from build123d import *

# Parameters (mm, degrees)
SKETCH2_R                 = 2.5
BOSS_EXTRUDE1_DEPTH       = 18
FILLET3_R                 = 1
BOSS_EXTRUDE2_START       = -1
SKETCH5_R                 = 3.75
SKETCH5_R_2               = 2.5
BOSS_EXTRUDE2_DEPTH       = 1
F_1_0MM_DOWEL_HOLE1_D     = 4
F_1_0MM_DOWEL_HOLE1_DEPTH = 13.785898385
F_1_0MM_DOWEL_HOLE1_TIP   = 3.464101615


with BuildPart() as part:
    # Sketch2 → Boss-Extrude1 (new body)
    with BuildSketch(Plane(origin=(0, 0, 0), x_dir=(1, 0, 0), z_dir=(0, 1, 0))):
        with Locations(Location((0, 0, 0), (0, 0, 270))):
            Circle(SKETCH2_R)
    extrude(amount=BOSS_EXTRUDE1_DEPTH)

    # Fillet3
    fillet3_edges = [part.edges().sort_by_distance(p)[0] for p in [
        (0, 0, -2.5),
    ]]
    fillet(fillet3_edges, radius=FILLET3_R)

    # Sketch5 → Boss-Extrude2 (add)
    with BuildSketch(Plane(origin=(0, 18, 0), x_dir=(1, 0, 0), z_dir=(0, 1, 0)).offset(BOSS_EXTRUDE2_START)):
        with Locations(Location((0, 0, 0), (0, 0, 270))):
            Circle(SKETCH5_R)
        with Locations(Location((0, 0, 0), (0, 0, 270))):
            Circle(SKETCH5_R_2, mode=Mode.SUBTRACT)
    extrude(amount=BOSS_EXTRUDE2_DEPTH)

    # Ø1.0mm Dowel Hole1
    with Locations(Plane(origin=(0, 18, 0), x_dir=(1, 0, 0), z_dir=(0, 1, 0))):
        with Locations((0, 0)):
            Hole(F_1_0MM_DOWEL_HOLE1_D / 2, depth=F_1_0MM_DOWEL_HOLE1_DEPTH)
            with Locations((0, 0, -(F_1_0MM_DOWEL_HOLE1_DEPTH + F_1_0MM_DOWEL_HOLE1_TIP / 2))):  # 60° drill point
                Cone(0, F_1_0MM_DOWEL_HOLE1_D / 2, F_1_0MM_DOWEL_HOLE1_TIP, mode=Mode.SUBTRACT)


solid = part.part
Check sheet for the modelled part. Datum: model origin and axes. Units: mm. A direction names the side the tool comes from. Coordinates: 2 decimals unless noted, no trailing zeros. Loops run counter-clockwise (first coordinate to the right, second up) from the corner with the lowest first, then second, coordinate; pieces in that order, holes last. Notation, with made-up numbers: (15.25, -6.75) -> (56.25, -6.75) arc R24 cw to (56.25, 14.25) -> close; hole circle Ø10 at (84.25, -13). An arc over 180 degrees is marked (long way). Write item = value, one per line. Start each with the question number.
1. Draft check along Z on faces 3 (the cylindrical face through (0.165, 17.493, -3.746)), 4 (the flat face through (0, 0, 0)), 5 (the cylindrical face through (0, 11, 2)). Enter one of: released by +Z, released by -Z, zero draft, split by the parting line, or undercut.
2. Tool access check on faces 1 (the flat face through (3, 17, 0)), 2 (the flat face through (-2, 18, 2)). Record the directions out of +Z, -Z, +X, -X, +Y, -Y that give a thin tool (end or side, any length) a straight path to the whole face; none if there is none.
3. Section check A-A on z = 3. Record the cut outline in (x, y).
4. Material ranges on line 1 (Y direction, x = 2.5, z = 2.25); line 2 (X direction, y = 2.75, z = 0.5); line 3 (Z direction, x = 1.5, y = 6.5), recorded low to high.
5. Section check B-B on y = 7.25. Record the cut outline in (x, z), then the cut area to 3 significant figures.
6. Section check C-C on y = 2.75. Record the cut outline in (x, z).
7. Depth check by flat-ended pin: P1, Ø1.5, axis at x = 0, y = 4.5, coming from the +Z side; P2, Ø3.5, axis at x = 0, z = 0, coming from the +Y side; P3, Ø3, axis at y = 7, z = 2, coming from the +X side. Enter the tip coordinate at first touch or a pass-through.
Responses:
q1.face_3 = split by the parting line
q1.face_4 = zero draft
q1.face_5 = undercut
q2.face_1 = -Y
q2.face_2 = +Z, -Z, +X, -X, +Y
q3.outline = (-2.25, 17) -> (2.25, 17) -> (2.25, 18) -> (-2.25, 18) -> close
q4.line_1 = 17 to 18
q4.line_2 = -2.45 to -1.04, 1.04 to 2.45
q4.line_3 = -2 to -1.32, 1.32 to 2
q5.outline = circle Ø5 at (0, 0); hole circle Ø4 at (0, 0)
q5.area = 7.07 mm2
q6.outline = circle Ø5 at (0, 0); hole circle Ø2.31 at (0, 0)
q7.P1 = 2.5
q7.P2 = 3.78
q7.P3 = 2.45
